The drawing under review shows one solid part. Ordinate dimensions are in mm from its lowest x, y, z. Coordinates: 2 decimals unless noted, no trailing zeros. Order: outer loops, then holes, each group sorted by start corner. A loop starts at its lowest first (then second) coordinate and runs counter-clockwise, first axis right, second up. Notation, with made-up numbers: (57.25, 50.5) -> (110.25, 50.5) arc R20 cw to (110.25, 86.5) -> close; hole circle Ø11 at (40.25, 64). An arc over 180 degrees is marked (long way). Use one line per item in the form item = value.
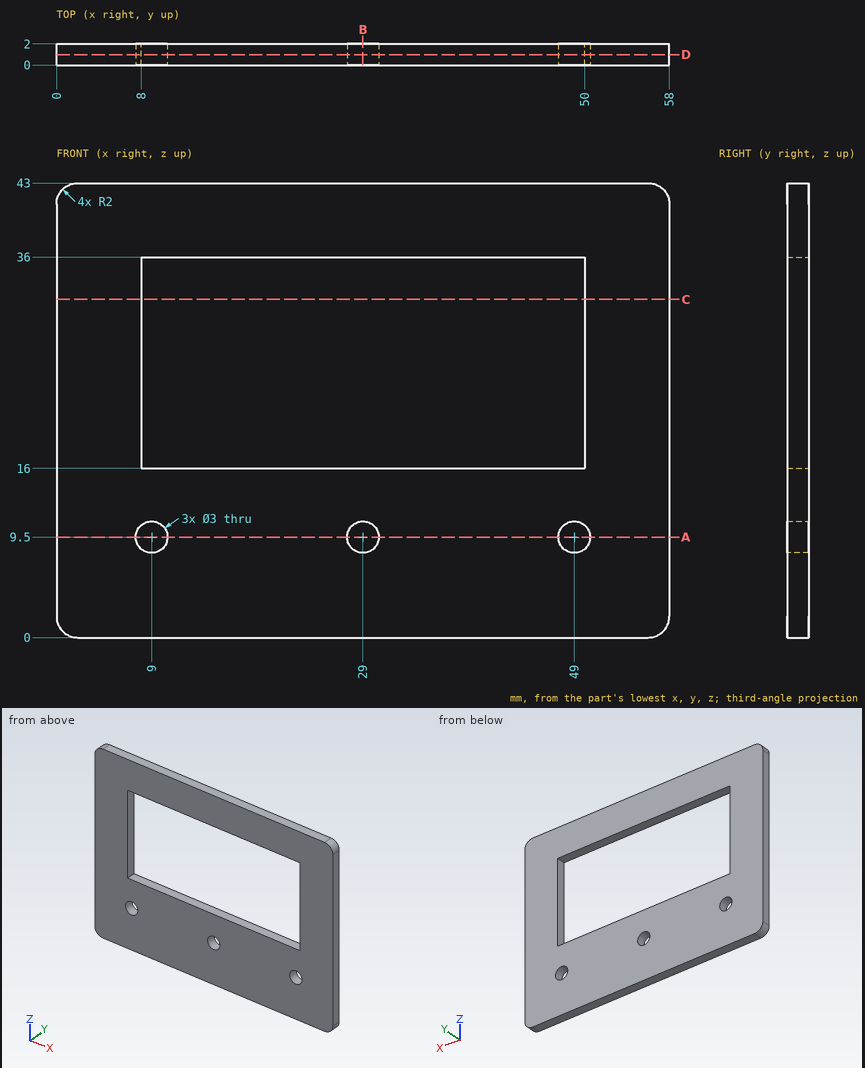
Item 1: We need section B-B (x = 29). Write out the cut boundary in (y, z).
Results found:
outline = (0, 0) -> (2, 0) -> (2, 8) -> (0, 8) -> close; (0, 11) -> (2, 11) -> (2, 16) -> (0, 16) -> close; (0, 36) -> (2, 36) -> (2, 43) -> (0, 43) -> close
Item 2: Clearance check with a flat-ended pin moving along its axis: pin 1 (12 mm diameter, centred on x = 38.5, z = 25.5, fed in from +Y). State where the tip first meets the part, or that it passes through.
Results found:
pin_1 = through
Item 3: To check wall thickness, follow L1, parallel to X at y = 1.5, z = 9.5; L2, parallel to Z at x = 20.5, y = 0.7; L3, parallel to X at y = 1, z = 31.5. State the ranges of each line that lie inside material, in increasing order. Write a range as from..to.
Results found:
L1 = 0..7.5, 10.5..27.5, 30.5..47.5, 50.5..58
L2 = 0..16, 36..43
L3 = 0..8, 50..58
Item 4: We need section D-D (y = 1). Write out the cut boundary in (x, z), plus the area to 3 significant figures.
Results found:
outline = (0, 2) arc R2 ccw to (2, 0) -> (56, 0) arc R2 ccw to (58, 2) -> (58, 41) arc R2 ccw to (56, 43) -> (2, 43) arc R2 ccw to (0, 41) -> close; hole circle Ø3 at (9, 9.5); hole (8, 16) -> (50, 16) -> (50, 36) -> (8, 36) -> close; hole circle Ø3 at (29, 9.5); hole circle Ø3 at (49, 9.5)
area = 1,630 mm²
Item 5: We need section C-C (z = 32). Write out the cut boundary in (x, y), plus the area to 3 significant figures.
Results found:
outline = (0, 0) -> (8, 0) -> (8, 2) -> (0, 2) -> close; (50, 0) -> (58, 0) -> (58, 2) -> (50, 2) -> close
area = 32.0 mm²
Item 6: We need section A-A (z = 9.5). Write out the cut boundary in (x, y), plus the area to 3 significant figures.
Results found:
outline = (0, 0) -> (7.5, 0) -> (7.5, 2) -> (0, 2) -> close; (10.5, 0) -> (27.5, 0) -> (27.5, 2) -> (10.5, 2) -> close; (30.5, 0) -> (47.5, 0) -> (47.5, 2) -> (30.5, 2) -> close; (50.5, 0) -> (58, 0) -> (58, 2) -> (50.5, 2) -> close
area = 98.0 mm²
